Read the model definition and answer for the solid it produces. Units are mm, in the model's axes. A direction names the side the tool comes from. Give positions to 0.01 mm unless a question says otherwise; leave off trailing zeros. Loops run counter-clockwise (first coordinate to the right, second up) from the corner with the lowest first, then second, coordinate; pieces in that order, holes last. Notation, with made-up numbers: (45.25, 74) - (64.25, 74) arc R24 cw to (64.25, 97) - close; hole circle Ø11 at (16.5, -33.75). An arc over 180 degrees is marked (long way). Write item = value, one per line.
```python
from build123d import *

# Parameters (mm, degrees)
F1_DEPTH = 19.05
F2_DEPTH = 5.08
F3_SIZE  = 6.35


with BuildPart() as f1:
    # F0 (on Top) → F1 (new body)
    with BuildSketch(Plane.XY):
        Polygon((12.7, 21.9970452561), (-12.7, 21.9970452561), (-25.4, 0), (-12.7, -21.9970452561), (12.7, -21.9970452561), (25.4, 0), align=None)
    extrude(amount=F1_DEPTH)

    # F0 (on Top) → F2 (join)
    with BuildSketch(Plane.XY):
        Polygon((-12.7, 21.9970452561), (-38.1, 21.9970452561), (-25.4, 0), align=None)
        Polygon((0, 43.9940905122), (-12.7, 21.9970452561), (12.7, 21.9970452561), align=None)
        Polygon((12.7, 21.9970452561), (-12.7, 21.9970452561), (-25.4, 0), (-12.7, -21.9970452561), (12.7, -21.9970452561), (25.4, 0), align=None)
        Polygon((-12.7, -21.9970452561), (-25.4, 0), (-38.1, -21.9970452561), align=None)
        Polygon((38.1, 21.9970452561), (12.7, 21.9970452561), (25.4, 0), align=None)
        Polygon((12.7, -21.9970452561), (-12.7, -21.9970452561), (0, -43.9940905122), align=None)
        Polygon((38.1, -21.9970452561), (25.4, 0), (12.7, -21.9970452561), align=None)
    extrude(amount=F2_DEPTH)

    # F3
    f3_edges = [f1.edges().sort_by_distance(p)[0] for p in [
        (0, -21.997045, 19.05),
        (19.05, -10.998523, 19.05),
        (19.05, 10.998523, 19.05),
        (0, 21.997045, 19.05),
        (-19.05, 10.998523, 19.05),
        (-19.05, -10.998523, 19.05),
    ]]
    chamfer(f3_edges, length=F3_SIZE)


solid = f1.part
```
1) A cutting plane is placed at D-D on x = 2. Determine the outline of the cut face in (y, z).
Output:
outline = (-40.53, 0) - (40.53, 0) - (40.53, 5.08) - (22, 5.08) - (22, 12.7) - (15.65, 19.05) - (-15.65, 19.05) - (-22, 12.7) - (-22, 5.08) - (-40.53, 5.08) - close
2) Find the intervals of material crossed by probe 1 along Y at (x, z) = (4, 10.5); probe 2 along Y at (x, z) = (28, 3); probe 3 along Y at (x, z) = (-26, 4.5), in increasing order.
Output:
probe_1 = -22 to 22
probe_2 = -22 to -4.5, 4.5 to 22
probe_3 = -22 to -1.04, 1.04 to 22
3) Each of these flat-tipped pins is pushed along its axis until it touches: P1, Ø6, axis at y = -16, z = 12.5, coming from the +X side; P2, Ø1.5, axis at x = 20, z = 3, coming from the +Y side; P3, Ø5, axis at y = -7, z = 16, coming from the -X side. Where does it stop, or does it pass through?
Output:
P1 = 17.89
P2 = 22
P3 = -20.78
4) A cutting plane is placed at B-B on y = 4.5. Determine the outline of the cut face in (x, z).
Output:
outline = (-28, 0) - (28, 0) - (28, 5.08) - (22.8, 5.08) - (22.8, 12.7) - (15.47, 19.05) - (-15.47, 19.05) - (-22.8, 12.7) - (-22.8, 5.08) - (-28, 5.08) - close
5) A cutting plane is placed at C-C on x = -21. Determine the outline of the cut face in (y, z), then the cut area to 3 significant figures.
Output:
outline = (-22, 0) - (22, 0) - (22, 5.08) - (7.62, 5.08) - (7.62, 12.7) - (0, 16.51) - (-7.62, 12.7) - (-7.62, 5.08) - (-22, 5.08) - close
area = 369 mm²
6) A tool of negligible diameter and unlimited length cuts with its end or side. For faces 1 (the face through (-18.961, 11.153, 8.837)), 2 (the face through (18.961, -11.153, 8.837)), 3 (the face through (-25, 21.997, 3)), 4 (the face through (-31.66, -10.84, 2.5)), from which of +Z, -Z, +X, -X, +Y, -Y can it reach the whole face along a straight path? Write none if from no direction.
Output:
face_1 = +Z, -X, +Y
face_2 = +Z, +X, -Y
face_3 = +Z, -Z, -X, +Y
face_4 = +Z, -Z, -X
7) The mould has two halves that part along Y. Classify faces 5 (the face through (31.839, -11.153, 2.504)), 6 (the face through (0, 31, 5.08)), 7 (the face through (0, 21.997, 9)): pulls with the +Y half, pulls with the -Y half, needs draft (parallel to the pull), parting line crosses it, or undercut.
Output:
face_5 = undercut
face_6 = needs draft
face_7 = pulls with the +Y half
8) A cutting plane is placed at A-A on z = 2. Determine the outline of the cut face in (x, y), then the cut area to 3 significant figures.
Output:
outline = (-38.1, -22) - (-12.7, -22) - (0, -43.99) - (12.7, -22) - (38.1, -22) - (25.4, 0) - (38.1, 22) - (12.7, 22) - (0, 43.99) - (-12.7, 22) - (-38.1, 22) - (-25.4, 0) - close
area = 3,350 mm²
